Geometry: final body of the model. Coordinates: model frame, mm. A direction names the side the tool comes from. Give positions to 0.01 mm unless a question says otherwise; leave off trailing zeros. Loops run counter-clockwise (first coordinate to the right, second up) from the corner with the lowest first, then second, coordinate; pieces in that order, holes last. Notation, with made-up numbers: (56, -40) - (84, -40) arc R10 cw to (84, -26) - close; hole circle Ø2 at (84.25, 3.25). An arc over 180 degrees is marked (long way). Use CSV: the item, a comma, the result in double quotes. Start each with the question number.
```python
from build123d import *

# Parameters (mm, degrees)
SKETCH1_W           = 49
SKETCH1_H           = 49
SKETCH1_R           = 15
SKETCH1_W_2         = 4
SKETCH1_H_2         = 5
SKETCH1_W_3         = 3
BOSS_EXTRUDE1_DEPTH = 3


with BuildPart() as part:
    # Sketch1 → Boss-Extrude1 (new body)
    with BuildSketch(Plane(origin=(0, 0, 0), x_dir=(1, 0, 0), z_dir=(0, 1, 0))):
        Rectangle(SKETCH1_W, SKETCH1_H)
        Circle(SKETCH1_R, mode=Mode.SUBTRACT)
        with Locations((-26.5, 0)):
            Rectangle(SKETCH1_W_2, SKETCH1_H_2)
        with Locations((26, 0)):
            Rectangle(SKETCH1_W_3, SKETCH1_H)
        Polygon((30.5, 27.5), (27.5, 27.5), (27.5, 24.5), (27.5, -24.5), (27.5, -27.5), (30.5, -27.5), align=None)
    extrude(amount=BOSS_EXTRUDE1_DEPTH)


solid = part.part
```
Item 1: Section B-B (z = 0). Output: boundary loops of the cut face in (x, y).
Item 2: Ray query, probe 1 along X at (y, z) = (0.95, 0); probe 2 along Z at (x, y) = (0, 1.3); probe 3 along X at (y, z) = (1.35, 21). Return the intervals inside material, ascending.
Item 3: Section D-D (z = -23.5). Output: boundary loops of the cut face in (x, y).
Item 4: Pin query (flat end, axial travel): pin 1 Ø12 at (x, z) = (-1.5, 6.5) entering from -Y; pin 2 Ø1.5 at (x, y) = (-27, 1) entering from +Z; pin 3 Ø1 at (x, y) = (7.5, 1) entering from +Z; pin 4 Ø1.5 at (y, z) = (1.5, 26.5) entering from -X. Return the tip coordinate at first contact, or that it passes through.
Item 5: Mould query, pull axis Z, two halves, no side actions, for faces 1 (the flat face through (1, 1, 24.5)), 2 (the flat face through (-24.5, 1, -13)), 3 (the flat face through (29, 1, -27.5)), 4 (the cylindrical face through (-14.985, 1.479, -0.66)). Classes: pulls with the +Z half, pulls with the -Z half, needs draft (parallel to the pull), parting line crosses it, or undercut.
Item 6: Section A-A (x = 0). Output: boundary loops of the cut face in (y, z), plus the area to 3 significant figures.
Item 7: Reachability of faces 5 (the flat face through (-27, 1, 2.5)), 6 (the flat face through (2, 1, -24.5)), 7 (the flat face through (29, 1, 27.5)) from +Z, -Z, +X, -X, +Y, -Y: full face, straight path, thin tool, end or side. Return the list, or none.
Item 8: Section C-C (y = 2.2). Output: boundary loops of the cut face in (x, z).
Outcome:
1,outline,"(-28.5, 0) - (-15, 0) - (-15, 3) - (-28.5, 3) - close; (15, 0) - (30.5, 0) - (30.5, 3) - (15, 3) - close"
2,probe 1,"x = -28.5 to -15, 15 to 30.5"
2,probe 2,"z = -24.5 to -15, 15 to 24.5"
2,probe 3,"x = -24.5 to 30.5"
3,outline,"(-24.5, 0) - (30.5, 0) - (30.5, 3) - (-24.5, 3) - close"
4,pin 1,"passes through"
4,pin 2,"stops at z = 2.5"
4,pin 3,"stops at z = 24.5"
4,pin 4,"stops at x = 27.5"
5,face 1,"pulls with the +Z half"
5,face 2,"needs draft"
5,face 3,"pulls with the -Z half"
5,face 4,"undercut"
6,outline,"(0, -24.5) - (3, -24.5) - (3, -15) - (0, -15) - close; (0, 15) - (3, 15) - (3, 24.5) - (0, 24.5) - close"
6,area,"57.0 mm2"
7,face 5,"+Z, -X, +Y, -Y"
7,face 6,"-Z, -X, +Y, -Y"
7,face 7,"+Z, +X, -X, +Y, -Y"
8,outline,"(-28.5, -2.5) - (-24.5, -2.5) - (-24.5, -24.5) - (27.5, -24.5) - (27.5, -27.5) - (30.5, -27.5) - (30.5, 27.5) - (27.5, 27.5) - (27.5, 24.5) - (-24.5, 24.5) - (-24.5, 2.5) - (-28.5, 2.5) - close; hole circle Ø30 at (0, 0)"
